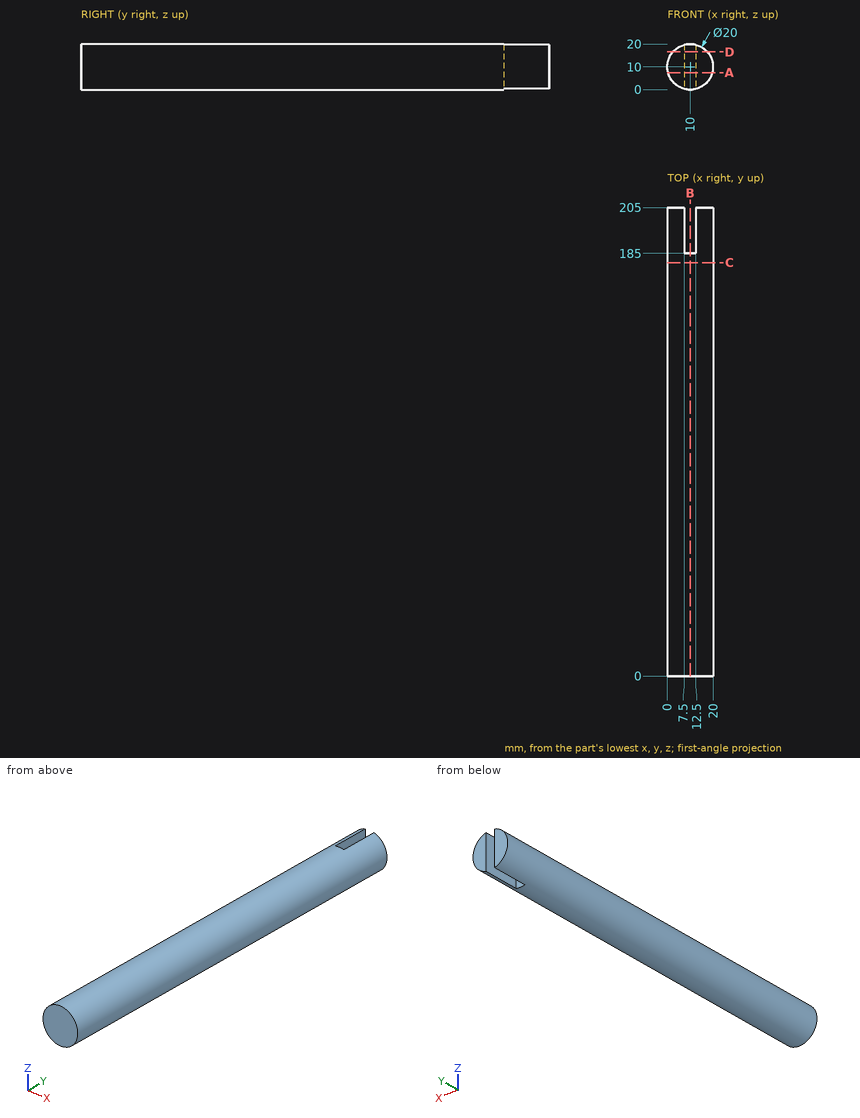
Input: dimensioned drawing with shaded views. Units: mm. Origin: part minimum x, y, z. Give positions to 0.01 mm unless a question says otherwise; leave off trailing zeros. Write each loop counter-clockwise with the first axis right and the second up, starting at its lowest first coordinate (ties: lowest second). Pieces come first, ordered by that corner, then holes. Notation, with made-up numbers: (60.5, -33.5) -> (115.5, -33.5) arc R22 ccw to (115.5, -5.5) -> close; hole circle Ø9 at (11.25, 48). An arc over 180 degrees is marked (long way). Answer as a JSON object with one key per item and string values.
1. Cut plane A-A on z = 7.5. Output: boundary loops of the cut face in (x, y), and give its area (3 significant figures).
Ans:
{"outline": "(0.32, 0) -> (19.68, 0) -> (19.68, 205) -> (12.5, 205) -> (12.5, 185) -> (7.5, 185) -> (7.5, 205) -> (0.32, 205) -> close", "area": "3,870 mm^2"}
2. Ray query, probe 1 along Z at (x, y) = (10.5, 74); probe 2 along Y at (x, z) = (10, 14.75); probe 3 along Z at (x, y) = (7.5, 142). Return the intervals inside material, ascending. Write a range as from..to.
Ans:
{"probe 1": "z = 0.01..19.99", "probe 2": "y = 0..185", "probe 3": "z = 0.32..19.68"}
3. Cut plane B-B on x = 10. Output: boundary loops of the cut face in (y, z), and give its area (3 significant figures).
Ans:
{"outline": "(0, 0) -> (185, 0) -> (185, 20) -> (0, 20) -> close", "area": "3,700 mm^2"}
4. Cut plane D-D on z = 16.5. Output: boundary loops of the cut face in (x, y).
Ans:
{"outline": "(2.4, 0) -> (17.6, 0) -> (17.6, 205) -> (12.5, 205) -> (12.5, 185) -> (7.5, 185) -> (7.5, 205) -> (2.4, 205) -> close"}
5. Contact query for flat-ended pins moving along their axis: pin 1 (3 mm diameter, centred on y = 25, z = 5, fed in from -X); pin 2 (2 mm diameter, centred on x = 12.5, y = 114, fed in from -Z); pin 3 (6 mm diameter, centred on y = 195.5, z = 6.5, fed in from -X). Output: stop coordinate, or through.
Ans:
{"pin 1": "stops at x = 0.63", "pin 2": "stops at z = 0.11", "pin 3": "stops at x = 0.01"}
6. Cut plane C-C on y = 181. Output: boundary loops of the cut face in (x, z), and give its area (3 significant figures).
Ans:
{"outline": "circle Ø20 at (10, 10)", "area": "314 mm^2"}
